```python
from build123d import *

# Parameters (mm, degrees)
BOSS_EXTRUDE1_DEPTH = 64
CUT_EXTRUDE1_DEPTH  = 64


with BuildPart() as part:
    # Sketch1 → Boss-Extrude1 (new body)
    with BuildSketch(Plane.XY):
        with BuildLine():
            Line((-201.08411215, 0), (-189.981308411, 22))
            Line((-189.981308411, 22), (-83.887850467, 22))
            Line((-83.887850467, 22), (-83.887850467, 117.401869159))
            Line((-83.887850467, 117.401869159), (-44.613332129, 117.401869159))
            Line((-44.613332129, 117.401869159), (-44.613332129, 63))
            Line((-44.613332129, 63), (-32, 63))
            ThreePointArc((-32, 63), (-22.308799202, 40.963993281), (0, 31.918417389))
            ThreePointArc((0, 31.918417389), (22.308799202, 40.963993281), (32, 63))
            Line((32, 63), (44.613332129, 63))
            Line((44.613332129, 63), (44.613332129, 117.401869159))
            Line((44.613332129, 117.401869159), (83.887850467, 117.401869159))
            Line((83.887850467, 117.401869159), (83.887850467, 22))
            Line((83.887850467, 22), (189.981308411, 22))
            Line((189.981308411, 22), (201.08411215, 0))
            Line((201.08411215, 0), (-201.08411215, 0))
        make_face()
    extrude(amount=BOSS_EXTRUDE1_DEPTH)

    # Sketch2 → Cut-Extrude1 (cut)
    with BuildSketch(Plane(origin=(0, 22, 0), x_dir=(1, 0, 0), z_dir=(0, 1, 0))):
        with BuildLine():
            Line((-171.985857657, -24.273514292), (-148.363703714, -24.273514292))
            ThreePointArc((-148.363703714, -24.273514292), (-140.075228646, -32.56198936), (-148.363703714, -40.850464428))
            Line((-148.363703714, -40.850464428), (-171.985857657, -40.850464428))
            ThreePointArc((-171.985857657, -40.850464428), (-180.274332725, -32.56198936), (-171.985857657, -24.273514292))
        make_face()
    cut_extrude1 = extrude(amount=-CUT_EXTRUDE1_DEPTH, mode=Mode.SUBTRACT)

    # Sketch5 → CBORE for M5 Hex Head Bolt1 (revolve, cut)
    with BuildSketch(Plane(origin=(-63.08411215, 0, 33.036059383), x_dir=(0, 0, -1), z_dir=(1, 0, 0))):
        Polygon((0, 0), (0, 135.708175881), (9.5, 130), (9.5, 12), (15, 12), (15, 0), align=None)
    cbore_for_m5_hex_head_bolt1 = revolve(axis=Axis((-63.08411215, -6.35, 33.036059383), (0, 1, 0)), mode=Mode.SUBTRACT)

    # Mirror1: Cut-Extrude1, CBORE for M5 Hex Head Bolt1 across plane
    add(cut_extrude1.mirror(Plane(origin=(0, 0, 0), x_dir=(0, 0, 1), z_dir=(1, 0, 0))), mode=Mode.SUBTRACT)
    add(cbore_for_m5_hex_head_bolt1.mirror(Plane(origin=(0, 0, 0), x_dir=(0, 0, 1), z_dir=(1, 0, 0))), mode=Mode.SUBTRACT)


solid = part.part
```
Model file for the job. Use its own axes, mm. A direction names the side the tool comes from. Coordinates: 2 decimals unless noted, no trailing zeros. Order: outer loops, then holes, each group sorted by start corner. A loop starts at its lowest first (then second) coordinate and runs counter-clockwise, first axis right, second up. Notation, with made-up numbers: M 10.5,16 L 59.5,16 A23 ccw 59.5,45 Z; hole C 81.5,-39.75 d5. An arc over 180 degrees is marked long. Answer as CSV lines item,"result".
(1) Band-saw the part on D-D, the plane y = 7. List the corners of the cut face in (x, z).
Geometry says:
outline,"M -197.55,0 L 197.55,0 L 197.55,64 L -197.55,64 Z; hole M -171.99,24.27 L -148.36,24.27 A8.29 ccw -148.36,40.85 L -171.99,40.85 A8.29 ccw Z; hole C -63.08,33.04 d30; hole C 63.08,33.04 d30; hole M 148.36,24.27 L 171.99,24.27 A8.29 ccw 171.99,40.85 L 148.36,40.85 A8.29 ccw Z"
(2) Flat gauge pins, fed straight in: pin 1 (6.5 mm diameter, centred on x = -37, z = 42.5, fed in from +Y); pin 2 (15 mm diameter, centred on x = -63, z = 29, fed in from -Y); pin 3 (10 mm diameter, centred on x = 41, z = 41, fed in from +Y); pin 4 (10 mm diameter, centred on x = -23, z = 38, fed in from +Y). Where does each tip first touch, or does it go through?
Geometry says:
pin 1,"stops at y = 63"
pin 2,"stops at y = 12"
pin 3,"stops at y = 117.4"
pin 4,"stops at y = 48.4"
(3) Wall check: line 1 along Z through (x, y) = (62, 59); line 2 along X through (y, z) = (74.5, 21.5); line 3 along X through (y, z) = (19, 32). Give the ranges that are in metal, low to high.
Geometry says:
line 1,"z = 0 to 23.6, 42.47 to 64"
line 2,"x = -83.89 to -44.61, 44.61 to 83.89"
line 3,"x = -191.5 to -180.26, -140.09 to -72.53, -53.64 to 53.64, 72.53 to 140.09, 180.26 to 191.5"
(4) Band-saw the part on C-C, the plane z = 14.5. List the corners of the cut face in (x, y).
Geometry says:
outline,"M -201.08,0 L 201.08,0 L 189.98,22 L 83.89,22 L 83.89,117.4 L 44.61,117.4 L 44.61,63 L 32,63 A32 cw 0,31.92 A32 cw -32,63 L -44.61,63 L -44.61,117.4 L -83.89,117.4 L -83.89,22 L -189.98,22 Z"
(5) Band-saw the part on A-A, the plane x = -152. List the corners of the cut face in (y, z), then the cut area to 3 significant figures.
Geometry says:
outline,"M 0,0 L 22,0 L 22,24.27 L 0,24.27 Z; M 0,40.85 L 22,40.85 L 22,64 L 0,64 Z"
area,"1,040 mm2"
(6) Band-saw the part on B-B, the plane y = 36. List the corners of the cut face in (x, z), then the cut area to 3 significant figures.
Geometry says:
outline,"M -83.89,0 L -15.65,0 L -15.65,64 L -83.89,64 Z; M 15.65,0 L 83.89,0 L 83.89,64 L 15.65,64 Z; hole C -63.08,33.04 d19; hole C 63.08,33.04 d19"
area,"8,170 mm2"
(7) 3-axis set-ups, long thin cutter, end or side, ignore diameter. For faces 5 (the cylindrical face through (-180.272, 11.154, 32.744)), 6 (the flat face through (53, 12, 33)), 7 (the flat face through (-138, 22, 32)), 8 (the flat face through (83.888, 70, 32)): which of +Z, -Z, +X, -X, +Y, -Y reach the whole face in a straight line?
Geometry says:
face 5,"+Y, -Y"
face 6,"-Y"
face 7,"+Z, -Z, -X, +Y"
face 8,"+Z, -Z, +X, +Y"
(8) Pull direction X, two halves, no side cores. Call faces 1 (the flat face through (136, 22, 32)), 2 (the flat face through (38, 63, 32)), 3 (the flat face through (-195.61, 10.85, 31.55)), 4 (the flat face through (-38, 63, 32)): +X half, -X half, draft (parallel to the pull), parting line (faces both ways), or undercut.
Geometry says:
face 1,"draft"
face 2,"undercut"
face 3,"-X half"
face 4,"undercut"
